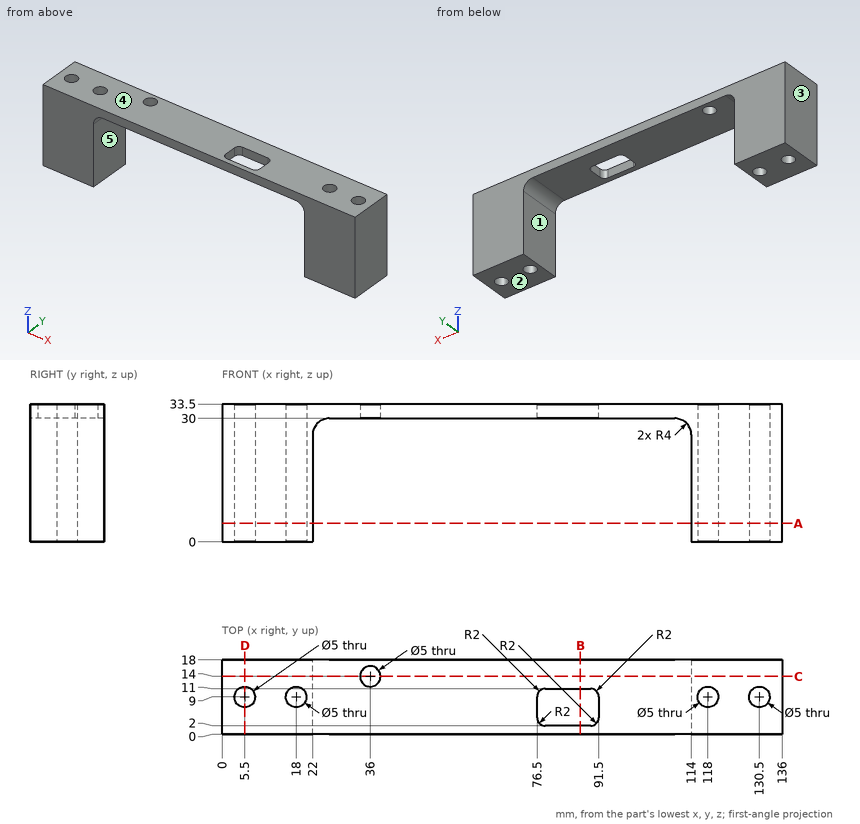
Design review of the part shown in the three views and the two pictorial views. Dimensions are in mm from the part's minimum x, y and z. A direction names the side the tool comes from. Round coordinates to 2 decimals unless told otherwise and drop trailing zeros. Order: outer loops, then holes, each group sorted by start corner. A loop starts at its lowest first (then second) coordinate and runs counter-clockwise, first axis right, second up. Notation, with made-up numbers: (79, 82.5) -> (110, 82.5) arc R27 ccw to (110, 112.5) -> close; hole circle Ø1 at (-25, -22). An arc over 180 degrees is marked (long way). Write item = value, one per line. Start each with the question number.
1) Tool access review of the marked faces 1 and 2: name each direction out of +Z, -Z, +X, -X, +Y, -Y from which nothing blocks a thin tool from reaching the whole face with its end or side.
2) Take a section at B-B on x = 87. State the section outline as (y, z) points, plus the area to 3 significant figures.
3) Take a section at A-A on z = 4.5. State the section outline as (x, y) points, plus the area to 3 significant figures.
4) Take a section at C-C on y = 14. State the section outline as (x, z) points, plus the area to 3 significant figures.
5) To check wall thickness, follow line 1 (X direction, y = 9, z = 24.5); line 2 (Y direction, x = 18, z = 19); line 3 (X direction, y = 15.75, z = 7). State the ranges of each line that lie inside material, in increasing order. Write a range as from..to.
6) The part is to be moulded in two halves that separate along X. For the marked faces 3, 4 and 5, say which applies: +X half, -X half, draft (parallel to the pull), parting line (faces both ways), or undercut.
7) Take a section at D-D on x = 5.5. State the section outline as (y, z) points.
8) Insertion check: pin 1 (1 mm diameter, centred on x = 31.5, y = 4.5, fed in from -Z). The pin has a flat end and moves straight along its axis. Give the tip position at first contact, or say it passes through.
Verdict:
q1.face_1 = -Z, +Y, -Y
q1.face_2 = -Z, +X, -X, +Y, -Y
q2.outline = (0, 30) -> (2, 30) -> (2, 33.5) -> (0, 33.5) -> close; (11, 30) -> (18, 30) -> (18, 33.5) -> (11, 33.5) -> close
q2.area = 31.5 mm2
q3.outline = (0, 0) -> (22, 0) -> (22, 18) -> (0, 18) -> close; (114, 0) -> (136, 0) -> (136, 18) -> (114, 18) -> close; hole circle Ø5 at (5.5, 9); hole circle Ø5 at (18, 9); hole circle Ø5 at (118, 9); hole circle Ø5 at (130.5, 9)
q3.area = 713 mm2
q4.outline = (0, 0) -> (22, 0) -> (22, 26) arc R4 cw to (26, 30) -> (33.5, 30) -> (33.5, 33.5) -> (0, 33.5) -> close; (38.5, 30) -> (110, 30) arc R4 cw to (114, 26) -> (114, 0) -> (136, 0) -> (136, 33.5) -> (38.5, 33.5) -> close
q4.area = 1,790 mm2
q5.line_1 = 0..3, 8..15.5, 20.5..22, 114..115.5, 120.5..128, 133..136
q5.line_2 = 0..6.5, 11.5..18
q5.line_3 = 0..22, 114..136
q6.face_3 = -X half
q6.face_4 = draft
q6.face_5 = undercut
q7.outline = (0, 0) -> (6.5, 0) -> (6.5, 33.5) -> (0, 33.5) -> close; (11.5, 0) -> (18, 0) -> (18, 33.5) -> (11.5, 33.5) -> close
q8.pin_1 = 30
